Could you check a few things on this model? Use its own coordinates, in mm. A direction names the side the tool comes from. Round coordinates to 2 decimals unless told otherwise and drop trailing zeros. Loops run counter-clockwise (first coordinate to the right, second up) from the corner with the lowest first, then second, coordinate; pieces in that order, holes last. Notation, with made-up numbers: (24, 3) -> (69, 3) arc R5 ccw to (69, 9) -> close; hole circle Ø4 at (23.5, 56.5). An arc over 180 degrees is marked (long way). One line per item, written item: value.
```python
from build123d import *

# Parameters (mm, degrees)
F0_R            = 31
F0_R_2          = 4.25
F1_DEPTH        = 5
F3_DEPTH        = 25
F3_COPIES_COUNT = 3
F4_R            = 2


# Not quite as in the source:
# - a pattern or mirror of a feature is missing from the dataset's text; its kind, count and spacing are read off the source's solid


with BuildPart() as f1:
    # F0 (on Top) → F1 (new body)
    with BuildSketch(Plane.XY):
        Circle(F0_R)
        Circle(F0_R_2, mode=Mode.SUBTRACT)
    extrude(amount=F1_DEPTH)

    # F2 (on face) → F3 (cut)
    with BuildSketch(Plane.XY.offset(5)):
        with BuildLine():
            ThreePointArc((1, 6.1694813396), (5.4126587737, 3.125), (5.8429275683, -2.218715266))
            Line((5.8429275683, -2.218715266), (25.599800796, -13.6253513424))
            ThreePointArc((25.599800796, -13.6253513424), (25.1147367097, 14.5), (1, 28.9827534924))
            Line((1, 28.9827534924), (1, 6.1694813396))
        make_face()
    f3 = extrude(amount=-F3_DEPTH, mode=Mode.SUBTRACT)

    # F3_copies: F3 ×3 about axis
    f3_copies_axis = Axis((0, 0, 0), (0, 0, 1))
    for i in range(1, F3_COPIES_COUNT):
        add(f3.rotate(f3_copies_axis, i * 360 / F3_COPIES_COUNT), mode=Mode.SUBTRACT)

    # F4
    f4_edges = [f1.edges().sort_by_distance(p)[0] for p in [
        (1, 6.169481, 2.5),
        (5.842928, -2.218715, 2.5),
        (25.599801, -13.625351, 2.5),
        (1, 28.982753, 2.5),
        (24.599801, -15.357402, 2.5),
        (-24.599801, -15.357402, 2.5),
        (4.842928, -3.950766, 2.5),
        (-4.842928, -3.950766, 2.5),
        (-25.599801, -13.625351, 2.5),
        (-1, 28.982753, 2.5),
        (-1, 6.169481, 2.5),
        (-5.842928, -2.218715, 2.5),
    ]]
    fillet(f4_edges, radius=F4_R)


solid = f1.part
```
(1) For pin 1 Ø2 at (y, z) = (-5, 1) entering from -X; pin 2 Ø1.5 at (x, z) = (12, 1.5) entering from +Y; pin 3 Ø2.5 at (y, z) = (18, 3) entering from -X, each with a flat end and sliding along its axis, tell me the tip position at first contact or that it passes through.
Results below:
pin 1: stops at x = -30.74
pin 2: stops at y = 28.89
pin 3: stops at x = -26.09
(2) Please list where these lines run through material, in increasing order: L1, parallel to X at y = 5.5, z = 4.7; L2, parallel to X at y = -11, z = 3.3; L3, parallel to Y at x = -10, z = 1.7.
Results below:
L1: x = -30.51 to -28.47, -2.97 to 2.97, 28.47 to 30.51
L2: x = -28.98 to -26.83, -21.05 to -17.05, 17.05 to 21.05, 26.83 to 28.98
L3: y = -29.34 to -27.22, -6.93 to -4.62, 27.22 to 29.34
(3) Imagine slicing it at C-C on z = 1.65. Write out the boundary of the cut face in (x, y), then the cut area to 3 significant figures.
Results below:
outline: circle Ø62 at (0, 0); hole (-26.57, -11.62) arc R2 ccw to (-23.74, -12.55) -> (-7.16, -2.98) arc R2 ccw to (-6.18, -0.94) arc R6.25 cw to (-2.27, 5.82) arc R2 ccw to (-1, 7.69) -> (-1, 26.83) arc R2 ccw to (-3.22, 28.82) arc R29 ccw to start; hole (-23.35, -17.2) arc R29 ccw to (23.35, -17.2) arc R2 ccw to (22.74, -14.28) -> (6.16, -4.71) arc R2 ccw to (3.91, -4.88) arc R6.25 cw to (-3.91, -4.88) arc R2 ccw to (-6.16, -4.71) -> (-22.74, -14.28) arc R2 ccw to start; hole circle Ø8.5 at (0, 0); hole (1, 7.69) arc R2 ccw to (2.27, 5.82) arc R6.25 cw to (6.18, -0.94) arc R2 ccw to (7.16, -2.98) -> (23.74, -12.55) arc R2 ccw to (26.57, -11.62) arc R29 ccw to (3.22, 28.82) arc R2 ccw to (1, 26.83) -> close
area: 588 mm²
(4) On a 3-axis mill with a long thin cutter (end or side, diameter ignored), from which of +Z, -Z, +X, -X, +Y, -Y can I reach the whole of each face in a straight line? I mean faces 5 (the face through (25.34, -12.726, 2.465)), 6 (the face through (-0.1, -4.4, 0)). Say none if no direction works.
Results below:
face 5: +Z, -Z
face 6: -Z, +X, -X, +Y, -Y
(5) Imagine slicing it at A-A on x = 0. Write out the boundary of the cut face in (y, z).
Results below:
outline: (-31, 0) -> (-29, 0) -> (-29, 5) -> (-31, 5) -> close; (-6.25, 0) -> (-4.25, 0) -> (-4.25, 5) -> (-6.25, 5) -> close; (4.25, 0) -> (31, 0) -> (31, 5) -> (4.25, 5) -> close
(6) Imagine slicing it at B-B on y = 0. Write out the boundary of the cut face in (x, z), then the cut area to 3 significant figures.
Results below:
outline: (-31, 0) -> (-29, 0) -> (-29, 5) -> (-31, 5) -> close; (-6.25, 0) -> (-4.25, 0) -> (-4.25, 5) -> (-6.25, 5) -> close; (4.25, 0) -> (6.25, 0) -> (6.25, 5) -> (4.25, 5) -> close; (29, 0) -> (31, 0) -> (31, 5) -> (29, 5) -> close
area: 40.0 mm²
(7) We'd pull the mould along X, two halves only. Please class faces 1 (the face through (-0.1, -4.4, 5)), 2 (the face through (5.021, -4.445, 2.465)), 3 (the face through (-5.442, 3.074, 2.535)), 4 (the face through (-4.036, 30.736, 2.465)): +X half, -X half, draft (parallel to the pull), parting line (faces both ways), or undercut.
Results below:
face 1: draft
face 2: undercut
face 3: undercut
face 4: parting line
(8) Imagine slicing it at D-D on y = 12.5. Write out the boundary of the cut face in (x, z).
Results below:
outline: (-28.37, 0) -> (-26.17, 0) -> (-26.17, 5) -> (-28.37, 5) -> close; (-1, 0) -> (1, 0) -> (1, 5) -> (-1, 5) -> close; (26.17, 0) -> (28.37, 0) -> (28.37, 5) -> (26.17, 5) -> close
